For this review, use the dimensioned drawing (mm, ordinates from the lowest corner) and the shaded views. A direction names the side the tool comes from. Round coordinates to 2 decimals unless told otherwise and drop trailing zeros. Order: outer loops, then holes, each group sorted by start corner. A loop starts at its lowest first (then second) coordinate and runs counter-clockwise, first axis right, second up. Notation, with made-up numbers: (-3.75, 12) - (19.25, 12) arc R29 cw to (19.25, 37) - close; hole circle Ø9 at (51.25, 34.5). An arc over 180 degrees is marked (long way). Write item = value, one per line.
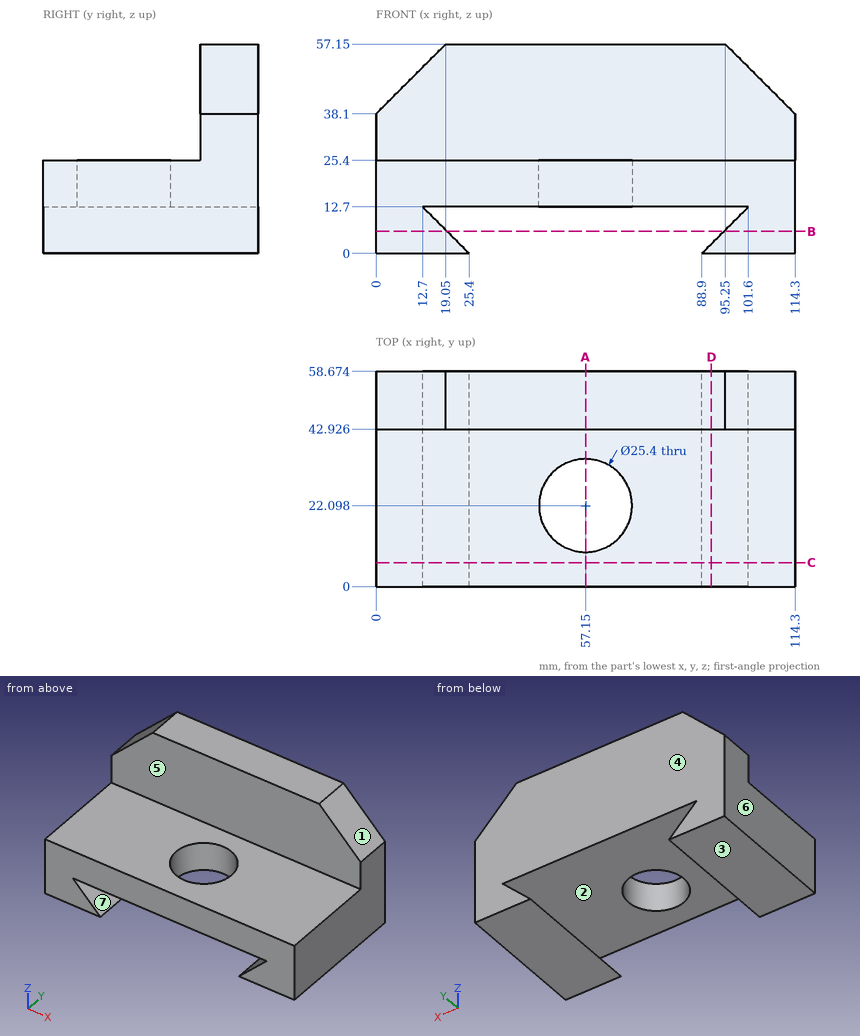
Item 1: Insertion check: P1, Ø1, axis at x = 97, y = 25, coming from the +Z side; P2, Ø3, axis at x = 23.5, z = 22.5, coming from the -Y side; P3, Ø23, axis at x = 57.15, y = 22.098, coming from the +Z side; P4, Ø12, axis at x = 43, z = 34.5, coming from the -Y side. Each pin has a flat end and moves straight along its axis. Give the tip position at first contact, or say it passes through.
Data:
P1 = 25.4
P2 = 0
P3 = through
P4 = 42.93
Item 2: Take a section at C-C, the plane y = 6.5. State the section outline as (x, z) points, and give its area (3 significant figures).
Data:
outline = (0, 0) - (25.4, 0) - (12.7, 12.7) - (101.6, 12.7) - (88.9, 0) - (114.3, 0) - (114.3, 25.4) - (0, 25.4) - close
area = 1,940 mm2
Item 3: Take a section at D-D, the plane x = 91.5. State the section outline as (y, z) points.
Data:
outline = (0, 0) - (58.67, 0) - (58.67, 2.6) - (0, 2.6) - close; (0, 12.7) - (58.67, 12.7) - (58.67, 57.15) - (42.93, 57.15) - (42.93, 25.4) - (0, 25.4) - close
Item 4: The part is to be moulded in two halves that separate along Z. For the marked faces 1, 2, 3 and 4, say which applies: +Z half, -Z half, draft (parallel to the pull), parting line (faces both ways), or undercut.
Data:
face_1 = +Z half
face_2 = undercut
face_3 = -Z half
face_4 = draft
Item 5: For line 1 along Y through (x, z) = (57.15, 19.5); line 2 along Y through (x, z) = (87, 31.5); line 3 along Z through (x, y) = (8, 11), list the stretches that pass through material, from the lowest coordinate up. Write a range as [from, to].
Data:
line_1 = [0, 9.4], [34.8, 58.67]
line_2 = [42.93, 58.67]
line_3 = [0, 25.4]
Item 6: Take a section at A-A, the plane x = 57.15. State the section outline as (y, z) points.
Data:
outline = (0, 12.7) - (9.4, 12.7) - (9.4, 25.4) - (0, 25.4) - close; (34.8, 12.7) - (58.67, 12.7) - (58.67, 57.15) - (42.93, 57.15) - (42.93, 25.4) - (34.8, 25.4) - close
Item 7: Take a section at B-B, the plane z = 6. State the section outline as (x, y) points.
Data:
outline = (0, 0) - (19.4, 0) - (19.4, 58.67) - (0, 58.67) - close; (94.9, 0) - (114.3, 0) - (114.3, 58.67) - (94.9, 58.67) - close
Item 8: For the marked faces 5, 6 and 7, list the 3-axis set-ups (+Z, -Z, +X, -X, +Y, -Y) from which the entire face can be reached by the end or side of a thin tool; tool diameter is ignored.
Data:
face_5 = +Z, +X, -X, -Y
face_6 = +Z, -Z, -X, +Y, -Y
face_7 = +Y, -Y
